Could you check a few things on this model? Use its own coordinates, in mm. A direction names the side the tool comes from. Coordinates: 2 decimals unless noted, no trailing zeros. Write each loop counter-clockwise with the first axis right and the second up, starting at its lowest first coordinate (ties: lowest second). Pieces come first, ordered by that corner, then holes.
Item 1: I want a section at B-B on y = 36.5. Please give me the cut outline in (x, z).
Item 2: If I drill on probe 1 along Y at (x, z) = (14.6, -7.5); probe 2 along Z at (x, y) = (12.75, 51); probe 3 along X at (y, z) = (16.5, -3.5), over which ranges is the centre line in solid material (lowest first)?
Item 3: Which directions (+Z, -Z, +X, -X, +Y, -Y) give clear straight access to the entire face, cutting with the end or side of a thin tool? Please do faces 1 (the flat face through (13.5, 44, -7)), 2 (the cylindrical face through (0.8, 11.6, -6.3)).
Item 4: I want a section at C-C on x = 3.75. Please give me the cut outline in (y, z), then the cut area to 3 significant figures.
Item 5: I want a section at A-A on z = -11.5. Please give me the cut outline in (x, y).
Item 6: I want a section at D-D on y = 57.5. Please give me the cut outline in (x, z).
Item 7: Thinking about a two-plate mould opening in X: for faces 3 (the flat face through (1.5, 44, -7)), 4 (the cylindrical face through (0.761, 78.987, -7.305)), 5 (the flat face through (7, 44, -1.5)), 6 (the flat face through (15, 44, -7)), which applies, +X half, -X half, draft (parallel to the pull), parting line (faces both ways), or undercut?
from build123d import *

# Parameters (mm, degrees)
SKETCH1_W           = 15
SKETCH1_H           = 15
SKETCH1_W_2         = 12
SKETCH1_H_2         = 12
EXTRUDE_THIN1_DEPTH = 90
SKETCH2_R           = 1.5
CUT_EXTRUDE1_DEPTH  = 16


with BuildPart() as part:
    # Sketch1 → Extrude-Thin1 (new body)
    with BuildSketch(Plane(origin=(0, 0, 0), x_dir=(1, 0, 0), z_dir=(0, 1, 0))):
        with Locations((7.5, 7.5)):
            Rectangle(SKETCH1_W, SKETCH1_H)
        with Locations((7.5, 7.5)):
            Rectangle(SKETCH1_W_2, SKETCH1_H_2, mode=Mode.SUBTRACT)
    extrude(amount=EXTRUDE_THIN1_DEPTH)

    # Sketch2 → Cut-Extrude1 (cut, through all)
    with BuildSketch(Plane(origin=(15, 0, 0), x_dir=(0, 0, -1), z_dir=(1, 0, 0))):
        with Locations((7.5, 12.5)):
            Circle(SKETCH2_R)
        with Locations((7.5, 32.5)):
            Circle(SKETCH2_R)
        with Locations((7.5, 57.5)):
            Circle(SKETCH2_R)
        with Locations((7.5, 77.5)):
            Circle(SKETCH2_R)
    extrude(amount=-CUT_EXTRUDE1_DEPTH, mode=Mode.SUBTRACT)


solid = part.part
Response values:
1. outline: (0, -15) - (15, -15) - (15, 0) - (0, 0) - close; hole (1.5, -13.5) - (13.5, -13.5) - (13.5, -1.5) - (1.5, -1.5) - close
2. probe 1: y = 0 to 11, 14 to 31, 34 to 56, 59 to 76, 79 to 90
2. probe 2: z = -15 to -13.5, -1.5 to 0
2. probe 3: x = 0 to 1.5, 13.5 to 15
3. face 1: +Y, -Y
3. face 2: +X, -X
4. outline: (0, -15) - (90, -15) - (90, -13.5) - (0, -13.5) - close; (0, -1.5) - (90, -1.5) - (90, 0) - (0, 0) - close
4. area: 270 mm2
5. outline: (0, 0) - (1.5, 0) - (1.5, 90) - (0, 90) - close; (13.5, 0) - (15, 0) - (15, 90) - (13.5, 90) - close
6. outline: (0, -15) - (15, -15) - (15, -9) - (13.5, -9) - (13.5, -13.5) - (1.5, -13.5) - (1.5, -9) - (0, -9) - close; (0, -6) - (1.5, -6) - (1.5, -1.5) - (13.5, -1.5) - (13.5, -6) - (15, -6) - (15, 0) - (0, 0) - close
7. face 3: undercut
7. face 4: draft
7. face 5: undercut
7. face 6: +X half
